```python
from build123d import *

# Parameters (mm, degrees)
BOSS_EXTRUDE3_DEPTH       = 12.7
BOSS_EXTRUDE3_DEPTH_BACK  = 88.9
SKETCH2_W                 = 21.40077
SKETCH2_H                 = 1.27
BOSS_EXTRUDE4_DEPTH       = 76.2
SKETCH3_W                 = 21.40077
SKETCH3_H                 = 1.905
BOSS_EXTRUDE5_DEPTH       = 12.7
SKETCH4_W                 = 21.40077
SKETCH4_H                 = 1.905
BOSS_EXTRUDE6_DEPTH       = 12.7
BOSS_EXTRUDE7_DEPTH       = 17.78
CUT_EXTRUDE1_DEPTH        = 3.556
BOSS_EXTRUDE8_DEPTH       = 17.78
CUT_EXTRUDE2_DEPTH        = 3.556
F_4_40_TAPPED_HOLE1_D     = 2.2606
F_4_40_TAPPED_HOLE1_DEPTH = 7.62
F_4_40_TAPPED_HOLE1_TIP   = 0.679152758
FILLET1_R                 = 2.794


with BuildPart() as part:
    # Sketch2 → Boss-Extrude3 (new, two sides: drawn at the far end of the back side and taken through both)
    with BuildSketch(Plane(origin=(0, 0, 0), x_dir=(1, 0, 0), z_dir=(0, 1, 0)).offset(-BOSS_EXTRUDE3_DEPTH_BACK)):
        with Locations((0, -11.335385)):
            Rectangle(SKETCH2_W, SKETCH2_H)
    extrude(amount=BOSS_EXTRUDE3_DEPTH + BOSS_EXTRUDE3_DEPTH_BACK)

    # Sketch2_3 → Boss-Extrude4 (add)
    with BuildSketch(Plane(origin=(0, 0, 0), x_dir=(1, 0, 0), z_dir=(0, 1, 0))):
        with BuildLine():
            ThreePointArc((0, -10.700385), (-3.462370633, -10.124733515), (-6.552209101, -8.459716014))
            Line((-6.552209101, -8.459716014), (-10.700385, -8.459716014))
            Line((-10.700385, -8.459716014), (-10.700385, -10.700385))
            Line((-10.700385, -10.700385), (0, -10.700385))
        make_face()
        with BuildLine():
            ThreePointArc((6.552209101, -8.459716014), (3.462370633, -10.124733515), (0, -10.700385))
            Line((0, -10.700385), (10.700385, -10.700385))
            Line((10.700385, -10.700385), (10.700385, -8.459716014))
            Line((10.700385, -8.459716014), (6.552209101, -8.459716014))
        make_face()
    extrude(amount=-BOSS_EXTRUDE4_DEPTH)

    # Sketch3 → Boss-Extrude5 (add)
    with BuildSketch(Plane(origin=(0, 0, 10.700385), x_dir=(-1, 0, 0), z_dir=(0, 0, -1))):
        with Locations((0, 0.9525)):
            Rectangle(SKETCH3_W, SKETCH3_H)
    extrude(amount=BOSS_EXTRUDE5_DEPTH)

    # Sketch4 → Boss-Extrude6 (add)
    with BuildSketch(Plane(origin=(0, 0, 10.700385), x_dir=(-1, 0, 0), z_dir=(0, 0, -1))):
        with Locations((0, -77.1525)):
            Rectangle(SKETCH4_W, SKETCH4_H)
    extrude(amount=BOSS_EXTRUDE6_DEPTH)

    # Sketch5 → Boss-Extrude7 (add)
    with BuildSketch(Plane(origin=(10.700385, 0, 0), x_dir=(0, 0, -1), z_dir=(1, 0, 0))):
        Polygon((-1.204354753, -3.186107507), (1.981752753, 0), (0.680653279, 0), (-1.971074087, -2.651727366), align=None)
    extrude(amount=-BOSS_EXTRUDE7_DEPTH)

    # Sketch5_4 → Cut-Extrude1 (cut)
    with BuildSketch(Plane(origin=(10.700385, 0, 0), x_dir=(0, 0, -1), z_dir=(1, 0, 0))):
        Polygon((-1.204354753, -3.186107507), (1.981752753, 0), (0.680653279, 0), (-1.971074087, -2.651727366), align=None)
    extrude(amount=-CUT_EXTRUDE1_DEPTH, mode=Mode.SUBTRACT)

    # Sketch6 → Boss-Extrude8 (add)
    with BuildSketch(Plane.ZY.offset(10.700385)):
        Polygon((0.530524719, -73.074012724), (-1.999615, -76.2), (-1.145153821, -76.2), (1.046780976, -73.49186486), align=None)
    extrude(amount=-BOSS_EXTRUDE8_DEPTH)

    # Sketch6_3 → Cut-Extrude2 (cut)
    with BuildSketch(Plane.ZY.offset(10.700385)):
        Polygon((0.530524719, -73.074012724), (-1.999615, -76.2), (-1.145153821, -76.2), (1.046780976, -73.49186486), align=None)
    extrude(amount=-CUT_EXTRUDE2_DEPTH, mode=Mode.SUBTRACT)

    # 4-40 Tapped Hole1
    with Locations(Plane(origin=(0, 0, 10.700385), x_dir=(-1, 0, 0), z_dir=(0, 0, -1))):
        with Locations((0, -83.82), (0, 7.62)):
            Hole(F_4_40_TAPPED_HOLE1_D / 2, depth=F_4_40_TAPPED_HOLE1_DEPTH)
            with Locations((0, 0, -(F_4_40_TAPPED_HOLE1_DEPTH + F_4_40_TAPPED_HOLE1_TIP / 2))):  # 118° drill point
                Cone(0, F_4_40_TAPPED_HOLE1_D / 2, F_4_40_TAPPED_HOLE1_TIP, mode=Mode.SUBTRACT)

    # Fillet1
    fillet1_edges = [part.edges().sort_by_distance(p)[0] for p in [
        (10.700385, 12.7, 11.335385),
        (-10.700385, -88.9, 11.335385),
        (10.700385, -88.9, 11.335385),
        (-10.700385, 12.7, 11.335385),
    ]]
    fillet(fillet1_edges, radius=FILLET1_R)


solid = part.part
```
Source: CAD feature listing. Evaluate the final solid. Frame: model axes, mm. A direction names the side the tool comes from. Give positions to 0.01 mm unless a question says otherwise; leave off trailing zeros. Loops run counter-clockwise (first coordinate to the right, second up) from the corner with the lowest first, then second, coordinate; pieces in that order, holes last. Notation, with made-up numbers: (38, -8) - (75, -8) arc R23 ccw to (75, 17) - close; hole circle Ø9 at (-8.5, 89). An arc over 180 degrees is marked (long way). Use CSV: the item, a comma, the result in double quotes. Start each with the question number.
1. Draft query along Y for faces 5 (the flat face through (10.7, -38, 9)), 6 (the cylindrical face through (9.904, -88.06, 11.326)), 7 (the flat face through (7.144, -1, 0)). Return one class per face: +Y half, -Y half, draft (parallel to the pull), parting line (faces both ways), or undercut.
2. Pin query (flat end, axial travel): pin 1 (10 mm diameter, centred on x = 5, y = -22.5, fed in from -Z); pin 2 (0.9 mm diameter, centred on y = -74.5, z = 0, fed in from -X); pin 3 (4 mm diameter, centred on x = -4.5, z = 4.5, fed in from -Y) (3 decimals). Return the tip coordinate at first contact, or that it passes through.
3. Section C-C (y = -26.5). Output: boundary loops of the cut face in (x, z), then the cut area to 3 significant figures.
4. Ray query, L1, parallel to Y at x = 0, z = 11.4; L2, parallel to Y at x = 1.25, z = 6.5 (3 decimals); L3, parallel to X at y = -83.82, z = 11.2. Return the intervals inside material, ascending.
5. Section D-D (x = 2.75). Output: boundary loops of the cut face in (y, z) (3 decimals), then the cut area to 3 significant figures.
6. Section B-B (y = -83.82). Output: boundary loops of the cut face in (x, z).
7. Section A-A (z = 5). Output: boundary loops of the cut face in (x, y) (3 decimals).
8. Reachability of faces 1 (the flat face through (0.132, -1.615, -0.366)), 2 (the flat face through (0, 6, 10.7)), 3 (the flat face through (0, 0, 4)), 4 (the flat face through (-7.08, -1, 0)) from +Z, -Z, +X, -X, +Y, -Y: full face, straight path, thin tool, end or side. Return the list, or none.
Response:
1,face 5,"draft"
1,face 6,"-Y half"
1,face 7,"undercut"
2,pin 1,"z = 8.46"
2,pin 2,"x = -7.14"
2,pin 3,"y = -78.105"
3,outline,"(-10.7, 8.46) - (-6.55, 8.46) arc R10.7 cw to (6.55, 8.46) - (10.7, 8.46) - (10.7, 11.97) - (-10.7, 11.97) - close"
3,area,"55.1 mm²"
4,L1,"-88.9 to -84.95, -82.69 to 6.49, 8.75 to 12.7"
4,L2,"-78.105 to -76.2, 0 to 1.905"
4,L3,"-10.7 to -1.13, 1.13 to 10.7"
5,outline,"(-88.9, 10.7) - (-78.105, 10.7) - (-78.105, -2) - (-76.2, -2) - (-73.074, 0.531) - (-73.492, 1.047) - (-76.2, -1.145) - (-76.2, 10.341) - (0, 10.341) - (0, -0.681) - (-2.652, 1.971) - (-3.186, 1.204) - (0, -1.982) - (0, -2) - (1.905, -2) - (1.905, 10.7) - (12.7, 10.7) - (12.7, 11.97) - (-88.9, 11.97) - close"
5,area,"211 mm²"
6,outline,"(-10.7, 10.7) - (-1.13, 10.7) - (-1.13, 11.97) - (-10.7, 11.97) - close; (1.13, 10.7) - (10.7, 10.7) - (10.7, 11.97) - (1.13, 11.97) - close"
7,outline,"(-10.7, -78.105) - (10.7, -78.105) - (10.7, -76.2) - (-10.7, -76.2) - close; (-10.7, 0) - (10.7, 0) - (10.7, 1.905) - (-10.7, 1.905) - close"
8,face 1,"-Z, +X, -X"
8,face 2,"-Z, +X, -X, +Y"
8,face 3,"none"
8,face 4,"-Z, -X"
